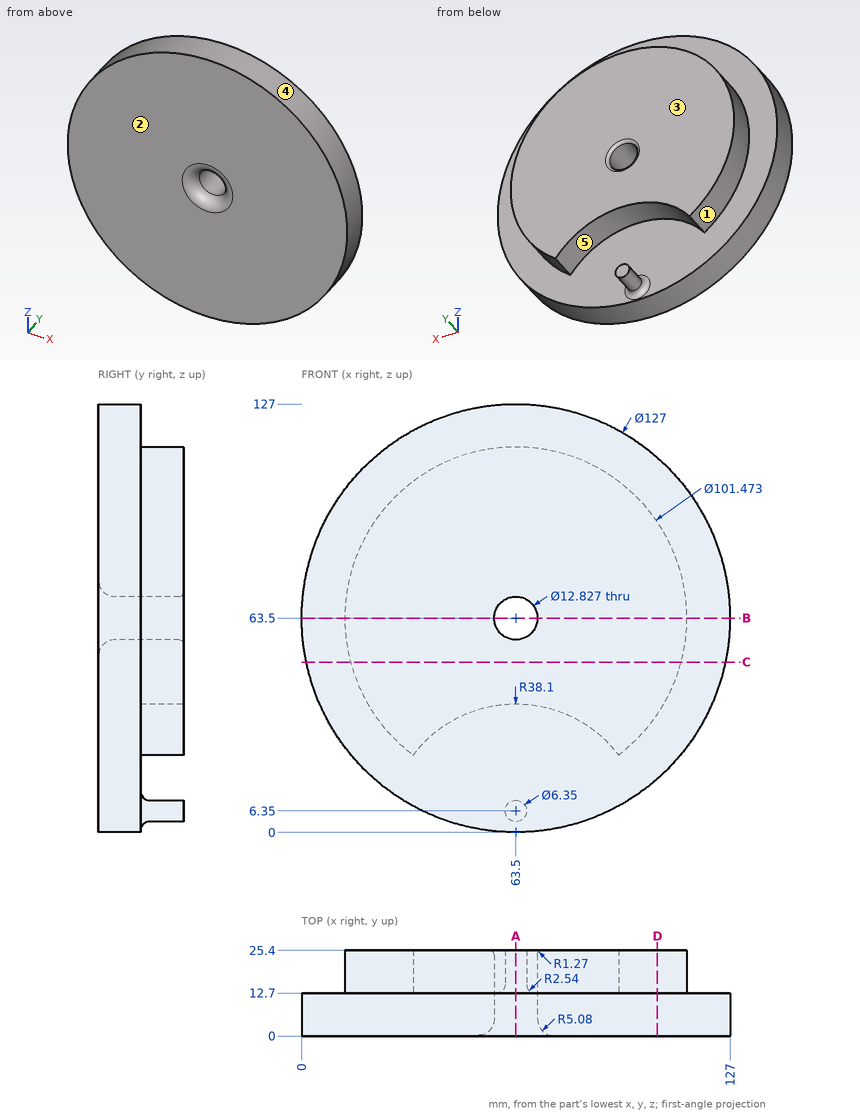
Print and shaded views of the part. All mm, measured from the part's lowest x, y and z. A direction names the side the tool comes from. Round coordinates to 2 decimals unless told otherwise and drop trailing zeros. Order: outer loops, then holes, each group sorted by start corner. A loop starts at its lowest first (then second) coordinate and runs counter-clockwise, first axis right, second up.
Q1. Wall check: L1, parallel to X at y = 3.75, z = 62; L2, parallel to X at y = 14, z = 63.5; L3, parallel to Y at x = 121.5, z = 49. Give the ranges that are in metal, low to high.
Q2. Two-plate mould, pull along X, no slides. Class the marked faces 3, 4 and 5: pulls with the +X half, pulls with the -X half, needs draft (parallel to the pull), parting line crosses it, or undercut.
Q3. Slice it at B-B (z = 63.5). Write the cut outline in (x, y), and give its area (3 significant figures).
Q4. Slice it at D-D (x = 105.5). Write the cut outline in (y, z).
Q5. Slice it at A-A (x = 63.5). Write the cut outline in (y, z) (1 decimal), and give its area (3 significant figures).
Q6. Drop flat-ended pins along their axis: pin 1 (5 mm diameter, centred on x = 21, z = 78, fed in from -Y); pin 2 (2 mm diameter, centred on x = 83.5, y = 22.5, fed in from +Z); pin 3 (5 mm diameter, centred on y = 16, z = 65, fed in from +X); pin 4 (2 mm diameter, centred on y = 22, z = 40, fed in from +X). Give the stop position or say it passes through.
Q7. Which spindle directions (+Z, -Z, +X, -X, +Y, -Y) get a long thin tool onto all of the face, cutting with end or side? Do the marked faces 1 and 2. Say none if no direction does.
Q8. Slice it at C-C (z = 50.5). Write the cut outline in (x, y).
Results below:
1. L1: x = 0.02 to 57.08, 69.92 to 126.98
1. L2: x = 12.76 to 57.09, 69.91 to 114.24
1. L3: y = 0 to 12.7
2. face 3: needs draft
2. face 4: parting line crosses it
2. face 5: undercut
3. outline: (0, 0) - (52.01, 0) arc R5.08 ccw to (57.09, 5.08) - (57.09, 24.13) arc R1.27 ccw to (55.82, 25.4) - (12.76, 25.4) - (12.76, 12.7) - (0, 12.7) - close; (69.91, 5.08) arc R5.08 ccw to (74.99, 0) - (127, 0) - (127, 12.7) - (114.24, 12.7) - (114.24, 25.4) - (71.18, 25.4) arc R1.27 ccw to (69.91, 24.13) - close
3. area: 2,560 mm2
4. outline: (0, 15.87) - (12.7, 15.87) - (12.7, 35.04) - (25.4, 35.04) - (25.4, 91.96) - (12.7, 91.96) - (12.7, 111.13) - (0, 111.13) - close
5. outline: (0, 0) - (12.7, 0) - (12.7, 0.6) arc R2.5 cw to (15.2, 3.2) - (25.4, 3.2) - (25.4, 9.5) - (15.2, 9.5) arc R2.5 cw to (12.7, 12.1) - (12.7, 38.1) - (25.4, 38.1) - (25.4, 55.8) arc R1.3 ccw to (24.1, 57.1) - (5.1, 57.1) arc R5.1 ccw to (0, 52) - close; (0, 75) arc R5.1 ccw to (5.1, 69.9) - (24.1, 69.9) arc R1.3 ccw to (25.4, 71.2) - (25.4, 114.2) - (12.7, 114.2) - (12.7, 127) - (0, 127) - close
5. area: 2,330 mm2
6. pin 1: stops at y = 0
6. pin 2: stops at z = 110.54
6. pin 3: stops at x = 114.24
6. pin 4: stops at x = 108.97
7. face 1: +Y
7. face 2: +Z, -Z, +X, -X, -Y
8. outline: (1.34, 0) - (125.66, 0) - (125.66, 12.7) - (112.54, 12.7) - (112.54, 25.4) - (14.46, 25.4) - (14.46, 12.7) - (1.34, 12.7) - close
